Build history of the part. All positions in model axes, mm. Coordinates: 2 decimals unless noted, no trailing zeros. Write each loop counter-clockwise with the first axis right and the second up, starting at its lowest first coordinate (ties: lowest second). Pieces come first, ordered by that corner, then holes. Notation, with made-up numbers: M 88.5,75.25 L 101.5,75.25 A22 cw 101.5,89.25 Z; hole C 10.5,72 d1. An arc over 180 degrees is marked long. Use CSV: the item, a comma, the result in double quotes. Start each with the question number.
Autodesk Inventor part; units mm, degrees
ref_plane "YZ Plane" through (0, 0, 0) normal (1, 0, 0) x (0, 1, 0)
ref_plane "XZ Plane" through (0, 0, 0) normal (0, 1, 0) x (-1, 0, 0)
ref_plane "XY Plane" through (0, 0, 0) normal (0, 0, 1) x (1, 0, 0)
sketch "Sketch1" plane through (0, 0, 0) normal (0, 0, 1) x (1, 0, 0)
  line L0 (0, 0) -> (0, 50)
  line L1 (0, 0) -> (62.5, 0)
  line L2 (62.5, 0) -> (62.5, 60)
  line L3 (62.5, 60) -> (52.5, 60)
  line L4 (52.5, 60) -> (52.5, 50)
  line L5 (52.5, 50) -> (0, 50)
  dimension "d0" = 125
  dimension "d1" = 60
  dimension "d2" = 50
  dimension "d3" = 10
revolve "Revolution1" add sketch "Sketch1" angle 360 about axis through (0, 0, 0) along (0, 1, 0)
fillet "Fillet1" radius 4.5 2 edges at (-62.5, 60, 0) (-52.5, 60, 0)
properties part number "Base"
1. Drill centre lines: line 1 along Z through (x, y) = (0, 51.4); line 2 along Y through (x, z) = (3, -43.5). Where is each one in solid material? Low to high. Write a range as from..to.
2. Flat gauge pins, fed straight in: pin 1 (3 mm diameter, centred on x = -37.5, y = 27, fed in from +Z); pin 2 (1 mm diameter, centred on y = 23.5, z = -42.5, fed in from +X); pin 3 (4 mm diameter, centred on y = 18, z = -37.5, fed in from +X). Where does each tip first touch, or does it go through?
3. Pull direction Z, two halves, no side cores. Call faces 1 (the cylindrical face through (50.076, 52.712, 15.77)), 2 (the flat face through (-1, 0, -1)), 3 (the flat face through (-1, 50, -1)), 4 (the cylindrical face through (-62.44, 28.14, -2.75)): pulls with the +Z half, pulls with the -Z half, needs draft (parallel to the pull), parting line crosses it, or undercut.
4. Slice it at B-B (z = 0). List the corners of the cut face in (x, y), and give its area (3 significant figures).
5. Slice it at D-D (y = 45). List the corners of the cut face in (x, z).
6. Slice it at C-C (y = 52). List the corners of the cut face in (x, z).
7. Slice it at A-A (x = 0). List the corners of the cut face in (y, z).
Established:
1,line 1,"z = -62.5..-52.5, 52.5..62.5"
1,line 2,"y = 0..50"
2,pin 1,"stops at z = 51.09"
2,pin 2,"stops at x = 46.28"
2,pin 3,"stops at x = 51.44"
3,face 1,"undercut"
3,face 2,"needs draft"
3,face 3,"undercut"
3,face 4,"parting line crosses it"
4,outline,"M -62.5,0 L 62.5,0 L 62.5,55.5 A4.5 ccw 58,60 L 57,60 A4.5 ccw 52.5,55.5 L 52.5,50 L -52.5,50 L -52.5,55.5 A4.5 ccw -57,60 L -58,60 A4.5 ccw -62.5,55.5 Z"
4,area,"6,430 mm2"
5,outline,"C 0,0 d125"
6,outline,"C 0,0 d125; hole C 0,0 d105"
7,outline,"M 0,-62.5 L 55.5,-62.5 A4.5 ccw 60,-58 L 60,-57 A4.5 ccw 55.5,-52.5 L 50,-52.5 L 50,52.5 L 55.5,52.5 A4.5 ccw 60,57 L 60,58 A4.5 ccw 55.5,62.5 L 0,62.5 Z"
